Source: three-view drawing plus pictorial views. Frame: mm from the lowest corner of the part. A direction names the side the tool comes from. Give positions to 0.01 mm unless a question says otherwise; leave off trailing zeros. Write each loop counter-clockwise with the first axis right and the second up, starting at its lowest first coordinate (ties: lowest second). Pieces come first, ordered by that corner, then holes.
Q1. Reachability of the marked faces 1, 2 and 3 from +Z, -Z, +X, -X, +Y, -Y: full face, straight path, thin tool, end or side. Return the list, or none.
Q2. Line query: L1, parallel to X at y = 0.75, z = 7.5; L2, parallel to X at y = 8.5, z = 9. Output: solid intervals per line, ascending.
Q3. Draft query along Z for the marked faces 4, 5 and 6. Return one class per face: pulls with the +Z half, pulls with the -Z half, needs draft (parallel to the pull), parting line crosses it, or undercut.
Q4. Cut plane B-B on z = 4.75. Return the cut outline in (x, y).
Q5. Cut plane C-C on y = 0.75. Return the cut outline in (x, z), plus the area to 3 significant figures.
Q6. Cut plane A-A on x = 8.25. Return the cut outline in (y, z).
Q7. Cut plane D-D on x = 2.25. Return the cut outline in (y, z), plus the area to 3 significant figures.
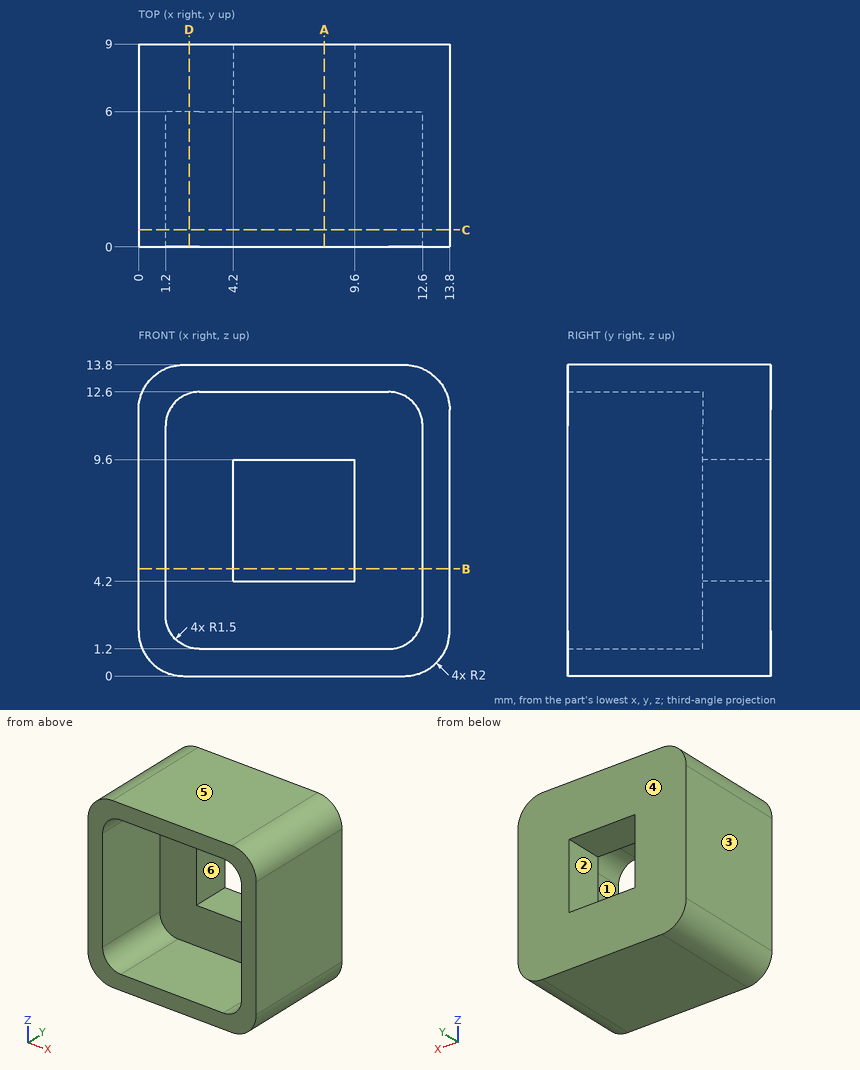
Data:
1. face 1: -Y
1. face 2: +Y, -Y
1. face 3: +Z, -Z, -X, +Y, -Y
2. L1: x = 0 to 1.2, 12.6 to 13.8
2. L2: x = 0 to 4.2, 9.6 to 13.8
3. face 4: needs draft
3. face 5: pulls with the +Z half
3. face 6: undercut
4. outline: (0, 0) - (1.2, 0) - (1.2, 6) - (4.2, 6) - (4.2, 9) - (0, 9) - close; (9.6, 6) - (12.6, 6) - (12.6, 0) - (13.8, 0) - (13.8, 9) - (9.6, 9) - close
5. outline: (0, 2) arc R2 ccw to (2, 0) - (11.8, 0) arc R2 ccw to (13.8, 2) - (13.8, 11.8) arc R2 ccw to (11.8, 13.8) - (2, 13.8) arc R2 ccw to (0, 11.8) - close; hole (1.2, 2.7) arc R1.5 ccw to (2.7, 1.2) - (11.1, 1.2) arc R1.5 ccw to (12.6, 2.7) - (12.6, 11.1) arc R1.5 ccw to (11.1, 12.6) - (2.7, 12.6) arc R1.5 ccw to (1.2, 11.1) - close
5. area: 59.0 mm2
6. outline: (0, 0) - (9, 0) - (9, 4.2) - (6, 4.2) - (6, 1.2) - (0, 1.2) - close; (0, 12.6) - (6, 12.6) - (6, 9.6) - (9, 9.6) - (9, 13.8) - (0, 13.8) - close
7. outline: (0, 0) - (9, 0) - (9, 13.8) - (0, 13.8) - (0, 12.53) - (6, 12.53) - (6, 1.27) - (0, 1.27) - close
7. area: 56.6 mm2
